from build123d import *

# Parameters (mm, degrees)
BOX_W           = 9
BOX_H           = 22
BOX_DEPTH       = 56.284271
POCKET077_DEPTH = 34.251
FILLET010_R     = 1
CHAMFER001_SIZE = 0.4


with BuildPart() as part:
    # Box → Box (join)
    with BuildSketch(Plane(origin=(-34.25, -11, -59.534271), x_dir=(1, 0, 0), z_dir=(0, 0, 1))):
        with Locations((4.5, 11)):
            Rectangle(BOX_W, BOX_H)
    extrude(amount=BOX_DEPTH)

    # Sketch136 → Pocket077 (cut, through all)
    with BuildSketch(Plane.YZ):
        with BuildLine():
            ThreePointArc((2.2, -13.25), (0, -11.05), (-2.2, -13.25))
            Line((-2.2, -13.25), (-2.2, -17.25))
            ThreePointArc((-2.2, -17.25), (0, -19.45), (2.2, -17.25))
            Line((2.2, -13.25), (2.2, -17.25))
        make_face()
    extrude(amount=-POCKET077_DEPTH, mode=Mode.SUBTRACT)

    # Sketch228 → Groove003 (revolve, cut)
    with BuildSketch(Plane.XZ):
        Polygon((-31.6, 0), (-31.6, -51.74899), (-28.6, -48.74899), (-28.6, -52.991631), (-33.1, -57.491631), (-36.1, -57.491631), (-36.1, -60.74899), (-19.6, -60.74899), (-19.6, 0), align=None)
    revolve(axis=Axis((0, 0, 0), (0, 0, 1)), mode=Mode.SUBTRACT)

    # Fillet010
    fillet010_edges = [part.edges().sort_by_distance(p)[0] for p in [
        (-32.734372, -11, -57.491631),
        (-28.815375, -11, -55.235201),
        (-32.734372, 11, -57.491631),
        (-28.815375, 11, -55.235201),
        (-26.4, 11, -50.87031),
        (-31.93682, 11, -3.25),
        (-31.93682, -11, -3.25),
    ]]
    fillet(fillet010_edges, radius=FILLET010_R)

    # Chamfer001
    chamfer001_edges = [part.edges().sort_by_distance(p)[0] for p in [
        (-34.25, 0, -57.491631),
        (-34.25, 10.707107, -57.198737),
        (-34.25, 11, -30.370815),
        (-34.25, 10.707107, -3.542893),
        (-34.25, 0, -3.25),
        (-34.25, -10.707107, -3.542893),
        (-34.25, -11, -30.370815),
        (-34.25, -10.707107, -57.198737),
        (-34.25, 0, -19.45),
        (-34.25, 2.2, -15.25),
        (-34.25, 0, -11.05),
        (-34.25, -2.2, -15.25),
    ]]
    chamfer(chamfer001_edges, length=CHAMFER001_SIZE)


with BuildPart() as part_1:
    # Body022028 placement: moved
    add(part.part.moved(Location((-3.125, 0, 854.79899))))


solid = part_1.part
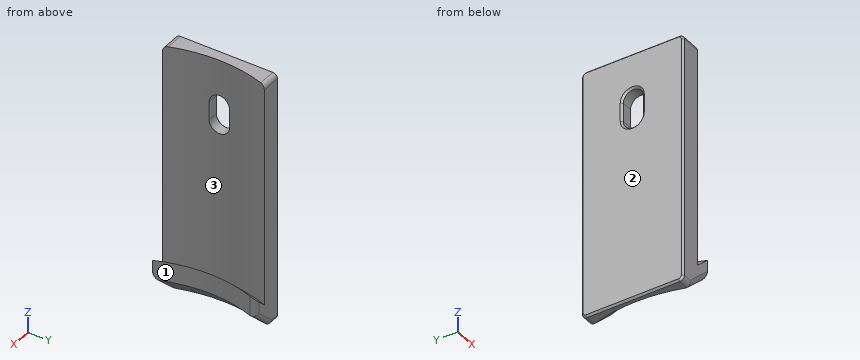
CAD build for the part. Positions are in the model's coordinates, mm. Face numbers are marked on the shaded views. Give positions to 0.01 mm unless a question says otherwise; leave off trailing zeros. Write each loop counter-clockwise with the first axis right and the second up, starting at its lowest first coordinate (ties: lowest second). Pieces come first, ordered by that corner, then holes. Notation, with made-up numbers: (-31.75, -9) - (25.25, -9) arc R25 ccw to (25.25, 26) - close; hole circle Ø1 at (-28.5, 15.25). An arc over 180 degrees is marked (long way). Answer as CSV lines item,"result".
Q1. Band-saw the part on B-B (z = 818.5). Give the cut face in (x, y) (3 decimals).
Result set:
outline,"(-37.375, -10.6) - (-36.975, -11) - (-32.749, -11) arc R31.6 cw to (-32.749, 11) - (-36.975, 11) - (-37.375, 10.6) - close"
Q2. Pull direction Y, two halves, no side cores. Call the marked faces 1, 2 and 3: released by +Y, released by -Y, zero draft, split by the parting line, or undercut.
Result set:
face 1,"undercut"
face 2,"zero draft"
face 3,"undercut"
Q3. Flat gauge pins, fed straight in: pin 1 Ø6 at (y, z) = (7, 820.5) entering from +X; pin 2 Ø3 at (x, z) = (-30.5, 841) entering from -Y; pin 3 Ø1 at (y, z) = (0, 805) entering from +X. Where does each tip first touch, or does it go through?
Result set:
pin 1,"x = -33.1"
pin 2,"through"
pin 3,"x = -31.72"
Q4. Band-saw the part on A-A (y = 0). Give the cut face in (x, z) (3 decimals), and give its area (3 significant figures).
Result set:
outline,"(-37.375, 797.707) - (-36.975, 797.307) - (-36.225, 797.307) - (-31.725, 801.807) - (-31.725, 806.05) - (-34.725, 803.05) - (-34.725, 835.349) - (-36.975, 835.349) - (-37.375, 834.949) - close; (-37.375, 844.149) - (-36.975, 843.749) - (-34.725, 843.749) - (-34.725, 851.549) - (-36.975, 851.549) - (-37.375, 851.149) - close"
area,"133 mm²"
Q5. Drill centre lines: line 1 (X direction, y = 5.25, z = 805.5) (3 decimals); line 2 (Z direction, x = -34, y = -4.25); line 3 (Z direction, x = -37, y = -6). Where is each one in solid material? Low to high. Write a range as from..to.
Result set:
line 1,"-37.375..-34.286, -31.798..-31.239"
line 2,"799.24..803.48"
line 3,"797.33..851.52"
